from build123d import *

# Parameters (mm, degrees)
ESQUISSE2_R                  = 250
BOSS_EXTRU_2_DEPTH           = 20
ESQUISSE3_R                  = 75
BOSS_EXTRU_3_DEPTH           = 30
R_P_TITION_CIRCULAIRE1_COUNT = 6


with BuildPart() as part:
    # Esquisse2 → Boss.-Extru.2 (new body)
    with BuildSketch(Plane(origin=(0, 0, 0), x_dir=(1, 0, 0), z_dir=(0, 1, 0))):
        with Locations(Location((0, 0, 0), (0, 0, 270))):
            Circle(ESQUISSE2_R)
    extrude(amount=BOSS_EXTRU_2_DEPTH)

    # Esquisse3 → Boss.-Extru.3 (add)
    with BuildSketch(Plane.XZ):
        with Locations(Location((0, 250, 0), (0, 0, 270))):
            Circle(ESQUISSE3_R)
    boss_extru_3 = extrude(amount=-BOSS_EXTRU_3_DEPTH)

    # Répétition circulaire1: Boss.-Extru.3 ×6 about axis
    r_p_tition_circulaire1_axis = Axis((0, 0, 0), (0, 1, 0))
    for i in range(1, R_P_TITION_CIRCULAIRE1_COUNT):
        add(boss_extru_3.rotate(r_p_tition_circulaire1_axis, i * 360 / R_P_TITION_CIRCULAIRE1_COUNT))


solid = part.part
Work out the finished part from the listing and answer in its coordinate system (mm). A direction names the side the tool comes from. Coordinates: 2 decimals unless noted, no trailing zeros. Loops run counter-clockwise (first coordinate to the right, second up) from the corner with the lowest first, then second, coordinate; pieces in that order, holes last. Notation, with made-up numbers: (-1, -26.75) -> (53, -26.75) arc R18 ccw to (53, -5.75) -> close; hole circle Ø9 at (22.25, 74). An arc over 180 degrees is marked (long way). Answer as CSV lines item,"result".
1) For faces 1 (the face through (4, 20, -3)), 2 (the face through (250, 10, 1)), determine the directions among +Z, -Z, +X, -X, +Y, -Y from which every point of the face is accessible in a straight line to the end or side of a thin tool.
A:
face 1,"+Y"
face 2,"+X, +Y, -Y"
2) The part is cut by section B-B (x = 0). Give the vertices of the cut face in (y, z).
A:
outline,"(0, -325) -> (30, -325) -> (30, -175) -> (20, -175) -> (20, 175) -> (30, 175) -> (30, 325) -> (0, 325) -> close"
3) The part is cut by section D-D (z = 250). Give the vertices of the cut face in (x, y), and give its area (3 significant figures).
A:
outline,"(-75, 0) -> (75, 0) -> (75, 30) -> (-75, 30) -> close"
area,"4,500 mm²"
4) Flat-ended cylindrical pins translate along their axes: pin 1 (1.5 mm diameter, centred on y = 10.5, z = 74, fed in from -X); pin 2 (1 mm diameter, centred on x = -17.5, z = -146.5, fed in from +Y); pin 3 (1.5 mm diameter, centred on y = 17, z = -242, fed in from +X). Find the tip coordinate at first contact, or state that the pin passes through.
A:
pin 1,"stops at x = -272.18"
pin 2,"stops at y = 20"
pin 3,"stops at x = 74.65"
5) For a pull along Z with two mould halves and no side action, classify faces 3 (the face through (-283.044, 18.123, -159.608)), 4 (the face through (-1, 30, -251)) as released by +Z, released by -Z, zero draft, split by the parting line, or undercut.
A:
face 3,"undercut"
face 4,"zero draft"
6) The part is cut by section C-C (y = 11). Give the vertices of the cut face in (x, z).
A:
outline,"(-243.84, -55.16) arc R75 ccw (long way) to (-169.69, -183.59) arc R250 ccw to (-74.15, -238.75) arc R75 ccw (long way) to (74.15, -238.75) arc R250 ccw to (169.69, -183.59) arc R75 ccw (long way) to (243.84, -55.16) arc R250 ccw to (243.84, 55.16) arc R75 ccw (long way) to (169.69, 183.59) arc R250 ccw to (74.15, 238.75) arc R75 ccw (long way) to (-74.15, 238.75) arc R250 ccw to (-169.69, 183.59) arc R75 ccw (long way) to (-243.84, 55.16) arc R250 ccw to start"
7) The part is cut by section A-A (z = 125). Give the vertices of the cut face in (x, y).
A:
outline,"(-291.51, 0) -> (291.51, 0) -> (291.51, 30) -> (141.51, 30) -> (141.51, 20) -> (-141.51, 20) -> (-141.51, 30) -> (-291.51, 30) -> close"
8) Straight lines are drawn through the part: probe 1 along X at (y, z) = (5.5, 185); probe 2 along Y at (x, z) = (28, 144.5); probe 3 along X at (y, z) = (8.5, 190.5). For each, find the intervals that lie inside material, in ascending order.
A:
probe 1,"x = -261.51 to -171.51, -168.15 to 168.15, 171.51 to 261.51"
probe 2,"y = 0 to 20"
probe 3,"x = -253.04 to -179.97, -161.89 to 161.89, 179.97 to 253.04"
